from build123d import *

# Parameters (mm, degrees)
EXTRUDE_1_DEPTH      = 1.65
EXTRUDE_1_DEPTH_BACK = 1.65
SKETCH_1_W           = 25
SKETCH_1_H           = 25
SKETCH_2_R           = 0.3
EXTRUDE_2_DEPTH      = 10


with BuildPart() as part:
    # Sketch 1 → Extrude 1 (new, two sides: drawn at the far end of the back side and taken through both)
    with BuildSketch(Plane(origin=(0, 0, 0), x_dir=(1, 0, 0), z_dir=(0, 1, 0)).offset(-EXTRUDE_1_DEPTH_BACK)):
        Rectangle(SKETCH_1_W, SKETCH_1_H)
    extrude(amount=EXTRUDE_1_DEPTH + EXTRUDE_1_DEPTH_BACK)

    # Sketch 2 → Extrude 2 (add)
    with BuildSketch(Plane.XY.offset(12.5)):
        with Locations(Location((-11, 0, 0), (0, 0, 180))):
            Circle(SKETCH_2_R)
        with Locations(Location((11, 0, 0), (0, 0, 180))):
            Circle(SKETCH_2_R)
    extrude(amount=EXTRUDE_2_DEPTH)


solid = part.part
Read the model definition and answer for the solid it produces. Units are mm, in the model's axes. Give positions to 0.01 mm unless a question says otherwise; leave off trailing zeros. Write each loop counter-clockwise with the first axis right and the second up, starting at its lowest first coordinate (ties: lowest second). Pieces come first, ordered by that corner, then holes. Notation, with made-up numbers: (31, 31) - (83, 31) arc R25 ccw to (83, 63) - close; hole circle Ø9 at (44, 81). An arc over 180 degrees is marked (long way). Return JSON: item names as keys, results as strings.
Q1. Consider line 1 along X through (y, z) = (-0.1, 16); line 2 along Z through (x, y) = (5.25, -1.15). Determine where each line is inside the solid, lowest interval first. Write a range as [from, to].
Reply:
{"line 1": "[-11.28, -10.72], [10.72, 11.28]", "line 2": "[-12.5, 12.5]"}
Q2. A cutting plane is placed at A-A, the plane z = 17. Determine the outline of the cut face in (x, y), and give its area (3 significant figures).
Reply:
{"outline": "circle Ø0.6 at (-11, 0); circle Ø0.6 at (11, 0)", "area": "0.565 mm²"}
Q3. A cutting plane is placed at C-C, the plane x = -4. Determine the outline of the cut face in (y, z), and give its area (3 significant figures).
Reply:
{"outline": "(-1.65, -12.5) - (1.65, -12.5) - (1.65, 12.5) - (-1.65, 12.5) - close", "area": "82.5 mm²"}
Q4. A cutting plane is placed at B-B, the plane y = -0.9. Determine the outline of the cut face in (x, z), and give its area (3 significant figures).
Reply:
{"outline": "(-12.5, -12.5) - (12.5, -12.5) - (12.5, 12.5) - (-12.5, 12.5) - close", "area": "625 mm²"}
